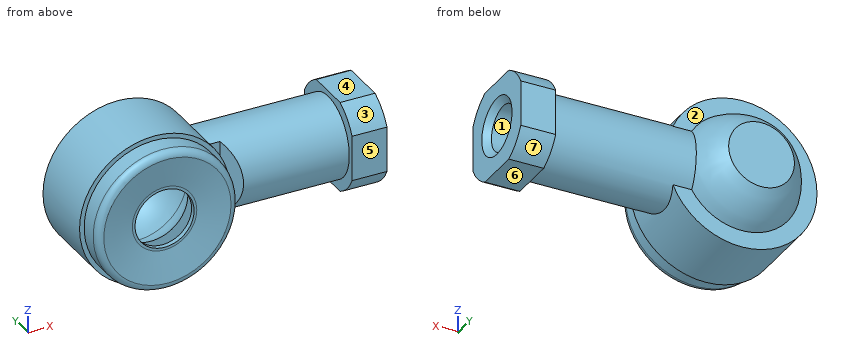
Autodesk Inventor part; units mm, degrees
ref_plane "IP1_XY" through (0, 16, 0) normal (0, 0, 1) x (1, 0, 0)
ref_plane "IP1_YZ" through (0, 16, 0) normal (1, 0, 0) x (0, 1, 0)
ref_plane "IP1_ZX" through (0, 16, 0) normal (0, 1, 0) x (0, 0, 1)
sketch "Sketch_2" plane through (0, 0, 0) normal (0, 0, 1) x (1, 0, 0)
  line L0 (43, 16) -> (0, 16)
  line L1 (0, 16) -> (0, 23.5)
  line L2 (0, 23.5) -> (36.5, 23.5)
  line L3 (36.5, 23.5) -> (36.5, 25.5)
  line L4 (36.5, 25.5) -> (43, 25.5)
  line L5 (43, 25.5) -> (43, 16)
  line L6 (43, 16) -> (0, 16)
revolve "Revolution1" add sketch "Sketch_2" angle 360 about axis through (43, 16, 0) along (1, 0, 0)
sketch "Sketch_16" plane through (0, 0, 0) normal (0, 0, 1) x (1, 0, 0)
  line L0 (-14, 12.5) -> (-14, 4.7)
  line L1 (-14, 4.7) -> (45.85, 4.7)
  line L2 (45.85, 4.7) -> (45.85, 27.3)
  line L3 (45.85, 27.3) -> (16.8094, 27.3)
  line L4 (16.8094, 27.3) -> (16.8094, 23.5)
  line L5 (16.8094, 23.5) -> (36.5, 23.5)
  line L6 (36.5, 23.5) -> (36.5, 24.5)
  line L7 (36.5, 24.5) -> (43, 24.5)
  line L8 (43, 24.5) -> (43, 7.5)
  line L9 (43, 7.5) -> (36.5, 7.5)
  line L10 (36.5, 7.5) -> (36.5, 8.5)
  line L11 (36.5, 8.5) -> (16.8094, 8.5)
  line L12 (16.8094, 8.5) -> (14.5, 12.5)
  line L13 (14.5, 12.5) -> (-14, 12.5)
extrude "Extrusion1" cut sketch "Sketch_16" along normal mid plane 38
sketch "Sketch_12" plane through (0, 0, 0) normal (0, 0, 1) x (1, 0, 0)
  line L0 (0, 9.5) -> (0, 28)
  line L1 (0, 28) -> (6.1238, 28)
  arc A0 (10.8825, 21) -> (6.1238, 28) centre (-4.0001, 16.0001) ccw
  line L2 (10.8825, 21) -> (14, 21)
  line L3 (14, 21) -> (14, 12.5)
  line L4 (14, 12.5) -> (12.825, 12.5)
  line L5 (12.825, 12.5) -> (12.825, 9.5)
  line L6 (12.825, 9.5) -> (0, 9.5)
  line L7 (0, 9.5) -> (0, 28)
revolve "Revolution2" add sketch "Sketch_12" angle 360 about axis through (0, 9.5, 0) along (0, -1, 0)
sketch "Sketch_13" plane through (0, 0, 0) normal (0, 0, 1) x (1, 0, 0)
  line L0 (9.525, 16) -> (-9.525, 16)
  arc A0 (9.525, 16) -> (-9.525, 16) centre (0, 16) ccw
  line L1 (9.525, 16) -> (-9.525, 16)
revolve "Revolution3" cut sketch "Sketch_13" angle 360 about axis through (9.525, 16, 0) along (1, 0, 0)
sketch "Sketch_14" plane through (0, 0, 0) normal (0, 0, 1) x (1, 0, 0)
  line L0 (0, 9.5) -> (0, 14.5)
  line L1 (0, 14.5) -> (10.6001, 14.5)
  line L2 (10.6001, 14.5) -> (10.6001, 9.5)
  line L3 (10.6001, 9.5) -> (0, 9.5)
  line L4 (0, 9.5) -> (0, 14.5)
revolve "Revolution4" cut sketch "Sketch_14" angle 360 about axis through (0, 9.5, 0) along (0, -1, 0)
sketch "Sketch_15" plane through (0, 0, 0) normal (0, 0, 1) x (1, 0, 0)
  line L0 (0, 9.5) -> (0, 14.5)
  line L1 (6.9624, 9.5) -> (10.6001, 9.5)
  line L2 (10.6001, 9.5) -> (10.6001, 14.5)
  line L3 (10.6001, 14.5) -> (9.4061, 14.5)
  arc A0 (6.9624, 9.5) -> (9.4061, 14.5) centre (0, 16) ccw
revolve "Revolution5" add sketch "Sketch_15" angle 360 about axis through (0, 9.5, 0) along (0, -1, 0)
sketch "Sketch_17" plane through (0, 0, 0) normal (0, 0, 1) x (1, 0, 0)
  line L0 (0, 4.5) -> (0, 12.5)
  line L1 (5.5, 5.4) -> (5.5, 4.5)
  line L2 (5.5, 4.5) -> (6, 4.5)
  line L3 (6, 4.5) -> (11.85, 3.4927)
  arc A0 (11.85, 3.4927) -> (13.15, 4.7927) centre (11.85, 4.7927) ccw
  line L4 (13.15, 4.7927) -> (13.15, 8)
  line L5 (13.15, 8) -> (14, 8)
  line L6 (14, 8) -> (14, 12.5)
  line L7 (14, 12.5) -> (12.825, 12.5)
  line L8 (12.825, 12.5) -> (12.825, 9.5)
  line L9 (12.825, 9.5) -> (12.25, 9.5)
  line L10 (12.25, 9.5) -> (12.25, 5.6927)
  arc A1 (10.95, 4.3927) -> (12.25, 5.6927) centre (10.95, 5.6927) ccw
  line L11 (10.95, 4.3927) -> (6, 5.4)
  line L12 (6, 5.4) -> (5.5, 5.4)
revolve "Revolution6" add sketch "Sketch_17" angle 360 about axis through (0, 4.5, 0) along (0, -1, 0)
sketch "Sketch8" plane through (43, 16, 0) normal (1, 0, 0) x (0, 0, -1)
  point P0 (0, 0)
hole "Hole1" at (43, 16, 0) direction (-1, 0, 0) diameter 8.376 depth 26.1765 tip angle 120 countersink diameter 10.729 countersink angle 90
sketch "Sketch_20" plane through (36.5, 0, 0) normal (1, 0, 0) x (0, 0, -1)
  line L0 (-12.75, 5.8) -> (12.75, 5.8)
  line L1 (12.75, 5.8) -> (12.75, 26.2)
  line L2 (12.75, 26.2) -> (-12.75, 26.2)
  line L3 (-12.75, 26.2) -> (-12.75, 5.8)
  line L4 (-8.5, 24.5) -> (-8.5, 7.5)
  line L5 (-8.5, 7.5) -> (8.5, 7.5)
  line L6 (8.5, 7.5) -> (8.5, 24.5)
  line L7 (8.5, 24.5) -> (-8.5, 24.5)
extrude "Extrusion2" cut sketch "Sketch_20" along normal blind 6.5
ref_plane "IP1_XY" through (0, 16, 0) normal (0, 0, 1) x (1, 0, 0)
ref_plane "IP1_YZ" through (0, 16, 0) normal (1, 0, 0) x (0, 1, 0)
ref_plane "IP1_ZX" through (0, 16, 0) normal (0, 1, 0) x (0, 0, 1)
properties part number "LHSA 10 Body1"
Design review of the part built by this model. Coordinates are the model's own, in mm. Face numbers are marked on the shaded views. A direction names the side the tool comes from. Give positions to 0.01 mm unless a question says otherwise; leave off trailing zeros. Order: outer loops, then holes, each group sorted by start corner. A loop starts at its lowest first (then second) coordinate and runs counter-clockwise, first axis right, second up. Notation, with made-up numbers: (19.25, -38.5) - (57.25, -38.5) arc R19 cw to (57.25, -12.5) - close; hole circle Ø4 at (17.5, 80.25). An arc over 180 degrees is marked (long way). Use a Markdown table: item, result. Add a question column.
(1) Wall thickness on probe 1 along Y at (x, z) = (25.75, 0); probe 2 along Z at (x, y) = (33.75, 16); probe 3 along X at (y, z) = (19.75, 7.75): over which ranges is each line inside the solid? List them lowest first. Write a range as [from, to].
(2) Clearance check with flat-ended pins moving along their axes: P1, Ø9.5, axis at y = 16, z = 0, coming from the +X side; P2, Ø1, axis at x = 26, y = 15.5, coming from the -Z side; P3, Ø10, axis at x = 14.5, z = -8.5, coming from the -Y side; P4, Ø5, axis at x = 41, y = 14.5, coming from the +Z side. State where each tip first meets the part, or that it passes through.
(3) Mouldability with a two-part tool opening along Y and no side actions: class the marked faces 1, 2 and 3 as +Y half, -Y half, draft (parallel to the pull), parting line (faces both ways), or undercut.
(4) Add section A-A on x = 39. Give the boundary of the cut face in (y, z), then the cut area to 3 significant figures.
(5) Add section B-B on x = 19. Give the boundary of the cut face in (y, z), then the cut area to 3 significant figures.
(6) Machinability: for the marked faces 4, 5, 6 and 7, which of the approach directions +Z, -Z, +X, -X, +Y, -Y give a long, thin tool a straight path to every point of the face, cutting with its end or side? Answer none if there is none.
Report:
| question | item | result |
|---|---|---|
| 1 | probe 1 | y = [8.5, 11.81], [20.19, 23.5] |
| 1 | probe 2 | z = [-7.5, -4.19], [4.19, 7.5] |
| 1 | probe 3 | x = [-11.66, -4.07], [4.07, 11.66], [36.5, 43] |
| 2 | P1 | stops at x = 42.39 |
| 2 | P2 | stops at z = -7.5 |
| 2 | P3 | stops at y = 3.49 |
| 2 | P4 | stops at z = 8.5 |
| 3 | face 1 | undercut |
| 3 | face 2 | +Y half |
| 3 | face 3 | -Y half |
| 4 | outline | (7.5, -4.24) arc R9.5 ccw to (11.76, -8.5) - (20.24, -8.5) arc R9.5 ccw to (24.5, -4.24) - (24.5, 4.24) arc R9.5 ccw to (20.24, 8.5) - (11.76, 8.5) arc R9.5 ccw to (7.5, 4.24) - close; hole circle Ø8.38 at (16, 0) |
| 4 | area | 206 mm² |
| 5 | outline | circle Ø15 at (16, 0); hole circle Ø8.38 at (16, 0) |
| 5 | area | 122 mm² |
| 6 | face 4 | +Z, +X, +Y, -Y |
| 6 | face 5 | +Z, -Z, +X, -Y |
| 6 | face 6 | -Z, +X, +Y, -Y |
| 6 | face 7 | -Z, +X, +Y |
